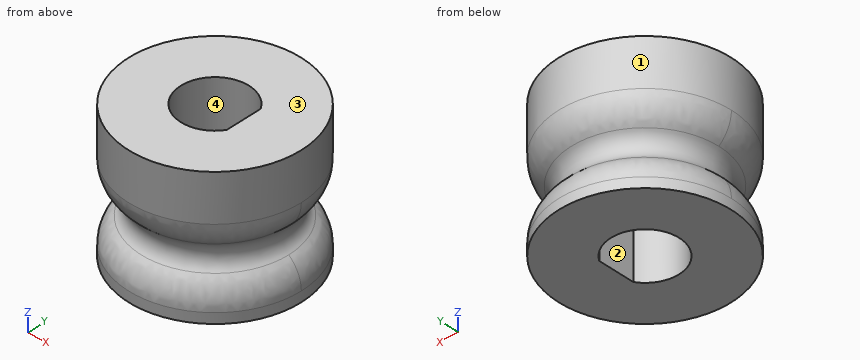
Autodesk Inventor part; units mm, degrees
ref_plane "YZ Plane" through (0, 0, 0) normal (1, 0, 0) x (0, 1, 0)
ref_plane "XZ Plane" through (0, 0, 0) normal (0, 1, 0) x (-1, 0, 0)
ref_plane "XY Plane" through (0, 0, 0) normal (0, 0, 1) x (1, 0, 0)
ref_plane "Work Plane1" through (0, 0, 0) normal (0, 0, 1) x (1, 0, 0)
sketch "Sketch1" plane through (0, 0, 0) normal (0, 0, 1) x (1, 0, 0)
  circle A0 centre (33.5, -2.875) radius 5.0649
  circle A1 centre (15, 1) radius 5.0649
  arc A2 (16.6873, 2.0738) -> (16.6873, -0.0738) centre (15, 1) ccw
  line L0 (16.6873, 2.0738) -> (16.6873, -0.0738)
  point P0 (0, 0)
  dimension "d4" = 4
extrude "Extrusion1" add sketch "Sketch1" along normal blind 8 contours A1
ref_plane "Work Plane2" through (23.5, 1, -28) normal (0, -1, 0) x (0, 0, 1)
sketch "Sketch2" plane through (23.5, 1, -28) normal (0, -1, 0) x (0, 0, 1)
  arc A0 (30.1735, -5.6017) -> (31.6642, -5.6017) centre (30.9188, -4.9351) ccw
  circle A1 centre (30.9188, 13.464) radius 1
  line L0 (26.4, 8.5) -> (37.6, 8.5)
  point P0 (28, 23.5)
revolve "Revolution1" cut sketch "Sketch2" angle 360 about axis through (15, 1, 0) along (0, 0, 1)
fillet "Fillet1" radius 2 4 edges at (15, -4.0649, 1.9239) (15, 6.0649, 1.9239) (15, -4.0649, 3.9137) (15, 6.0649, 3.9137)
properties part number "20_Cube_Insert_Lightsheet_FEPTube_Rotating_hollomotor_driver_v0"
Design review of the part built by this model. Coordinates are the model's own, in mm. Face numbers are marked on the shaded views. Give positions to 0.01 mm unless a question says otherwise; leave off trailing zeros. Order: outer loops, then holes, each group sorted by start corner. A loop starts at its lowest first (then second) coordinate and runs counter-clockwise, first axis right, second up.
1. Add section B-B, the plane z = 3. State the section outline as (x, y) points.
Solution:
outline: circle Ø7.93 at (15, 1); hole (16.69, -0.07) - (16.69, 2.07) arc R2 ccw (long way) to start
2. To check wall thickness, follow L1, parallel to Y at x = 15, z = 6; L2, parallel to Y at x = 16, z = 4.5; L3, parallel to X at y = 2.25, z = 3.75. State the ranges of each line that lie inside material, in increasing order.
Solution:
L1: y = -4.06 to -1, 3 to 6.06
L2: y = -3.82 to -0.73, 2.73 to 5.82
L3: x = 10.78 to 13.44, 16.56 to 19.22
3. Add section A-A, the plane z = 7. State the section outline as (x, y) points.
Solution:
outline: circle Ø10.13 at (15, 1); hole (16.69, -0.07) - (16.69, 2.07) arc R2 ccw (long way) to start
4. Mouldability with a two-part tool opening along Y and no side actions: class the marked faces 1, 2, 3 and 4 as +Y half, -Y half, draft (parallel to the pull), parting line (faces both ways), or undercut.
Solution:
face 1: parting line
face 2: undercut
face 3: draft
face 4: undercut
5. For pin 1 Ø4 at (x, z) = (15.5, 1.5) entering from -Y; pin 2 Ø2.5 at (y, z) = (0.5, 3) entering from -X; pin 3 Ø3 at (y, z) = (3.5, 2.5) entering from +X; pin 4 Ø4 at (x, z) = (12.5, 3) entering from +Y, all flat-tipped, find the tip position at first contact; note any pin that passes through.
Solution:
pin 1: stops at y = -4.06
pin 2: stops at x = 10.22
pin 3: stops at x = 19.67
pin 4: stops at y = 5.79
